from build123d import *

# Parameters (mm, degrees)
SKETCH1_W           = 60
SKETCH1_H           = 40
BOSS_EXTRUDE1_DEPTH = 10
SKETCH2_W           = 2.909575839
SKETCH2_H           = 3.168204802
CUT_EXTRUDE1_DEPTH  = 10
SKETCH3_W           = 61.747665015
SKETCH3_H           = 0.72949372
CUT_EXTRUDE2_DEPTH  = 2


with BuildPart() as part:
    # Sketch1 → Boss-Extrude1 (new body)
    with BuildSketch(Plane.XY):
        with Locations((1.914893617, 6.489361702)):
            Rectangle(SKETCH1_W, SKETCH1_H)
    extrude(amount=BOSS_EXTRUDE1_DEPTH)

    # Sketch2 → Cut-Extrude1 (cut)
    with BuildSketch(Plane.XY.offset(10)):
        with Locations((-13.721702382, 21.942442266)):
            Rectangle(SKETCH2_W, SKETCH2_H)
        with Locations((-23.721702382, 21.942442266)):
            Rectangle(SKETCH2_W, SKETCH2_H)
        with Locations((-3.721702382, 21.942442266)):
            Rectangle(SKETCH2_W, SKETCH2_H)
        with Locations((6.278297618, 21.942442266)):
            Rectangle(SKETCH2_W, SKETCH2_H)
        with Locations((16.278297619, 21.942442266)):
            Rectangle(SKETCH2_W, SKETCH2_H)
        with Locations((26.278297619, 21.942442266)):
            Rectangle(SKETCH2_W, SKETCH2_H)
        with Locations((-13.721702382, 11.942442266)):
            Rectangle(SKETCH2_W, SKETCH2_H)
        with Locations((-3.721702382, 11.942442266)):
            Rectangle(SKETCH2_W, SKETCH2_H)
        with Locations((6.278297618, 11.942442266)):
            Rectangle(SKETCH2_W, SKETCH2_H)
        with Locations((16.278297619, 11.942442266)):
            Rectangle(SKETCH2_W, SKETCH2_H)
        with Locations((26.278297619, 11.942442266)):
            Rectangle(SKETCH2_W, SKETCH2_H)
        with Locations((-13.721702382, 1.942442266)):
            Rectangle(SKETCH2_W, SKETCH2_H)
        with Locations((-3.721702382, 1.942442266)):
            Rectangle(SKETCH2_W, SKETCH2_H)
        with Locations((6.278297618, 1.942442266)):
            Rectangle(SKETCH2_W, SKETCH2_H)
        with Locations((16.278297619, 1.942442266)):
            Rectangle(SKETCH2_W, SKETCH2_H)
        with Locations((26.278297619, 1.942442266)):
            Rectangle(SKETCH2_W, SKETCH2_H)
        with Locations((-13.721702382, -8.057557734)):
            Rectangle(SKETCH2_W, SKETCH2_H)
        with Locations((-3.721702382, -8.057557734)):
            Rectangle(SKETCH2_W, SKETCH2_H)
        with Locations((6.278297618, -8.057557734)):
            Rectangle(SKETCH2_W, SKETCH2_H)
        with Locations((16.278297619, -8.057557734)):
            Rectangle(SKETCH2_W, SKETCH2_H)
        with Locations((26.278297619, -8.057557734)):
            Rectangle(SKETCH2_W, SKETCH2_H)
        with Locations((-23.721702382, 11.942442266)):
            Rectangle(SKETCH2_W, SKETCH2_H)
        with Locations((-23.721702382, 1.942442266)):
            Rectangle(SKETCH2_W, SKETCH2_H)
        with Locations((-23.721702382, -8.057557734)):
            Rectangle(SKETCH2_W, SKETCH2_H)
    extrude(amount=-CUT_EXTRUDE1_DEPTH, mode=Mode.SUBTRACT)

    # Sketch3 → Cut-Extrude2 (cut)
    with BuildSketch(Plane.XY.offset(10)):
        with Locations((1.945695922, 6.927829606)):
            Rectangle(SKETCH3_W, SKETCH3_H)
    extrude(amount=-CUT_EXTRUDE2_DEPTH, mode=Mode.SUBTRACT)


solid = part.part
Design review of the part built by this model. Coordinates are the model's own, in mm. A direction names the side the tool comes from. Give positions to 0.01 mm unless a question says otherwise; leave off trailing zeros. Order: outer loops, then holes, each group sorted by start corner. A loop starts at its lowest first (then second) coordinate and runs counter-clockwise, first axis right, second up. Notation, with made-up numbers: (-22.75, 30) - (-10.75, 30) arc R23 cw to (-10.75, 47) - close; hole circle Ø11 at (70.5, 52.25). An arc over 180 degrees is marked (long way). Use CSV: the item, a comma, the result in double quotes. Start each with the question number.
Q1. Take a section at C-C (z = 9). Count the separate pieces of the cut face and the enclosed holes in it, and give its area (4 significant figures).
Q2. Take a section at A-A (x = -24). State the section outline as (y, z) points, and give its area (3 significant figures).
Q3. For line 1 (Y direction, x = 5.5, z = 5.75); line 2 (Y direction, x = -21.5, z = 9); line 3 (Y direction, x = -14.5, z = 9), list the stretches that pass through material, from the lowest coordinate up.
Q4. Draft analysis for pull direction X (two halves, no side actions). For faces 3 (the face through (-28.085, 6, 5)), 4 (the face through (1, -3, 10)), 5 (the face through (16, 23.527, 5)), state which applies: pulls with the +X half, pulls with the -X half, needs draft (parallel to the pull), parting line crosses it, or undercut.
Q5. Take a section at B-B (y = 22.5). State the section outline as (x, z) points.
Q6. Machinability: for faces 1 (the face through (1, 17, 10)), 2 (the face through (-24, 0.358, 5)), which of the approach directions +Z, -Z, +X, -X, +Y, -Y give a long, thin tool a straight path to every point of the face, cutting with its end or side? Answer none if there is none.
Calculated:
1,separate pieces,"2"
1,enclosed holes,"24"
1,area,"2,135 mm²"
2,outline,"(-13.51, 0) - (-9.64, 0) - (-9.64, 10) - (-13.51, 10) - close; (-6.47, 0) - (0.36, 0) - (0.36, 10) - (-6.47, 10) - close; (3.53, 0) - (10.36, 0) - (10.36, 10) - (7.29, 10) - (7.29, 8) - (6.56, 8) - (6.56, 10) - (3.53, 10) - close; (13.53, 0) - (20.36, 0) - (20.36, 10) - (13.53, 10) - close; (23.53, 0) - (26.49, 0) - (26.49, 10) - (23.53, 10) - close"
2,area,"272 mm²"
3,line 1,"y = -13.51 to -9.64, -6.47 to 0.36, 3.53 to 10.36, 13.53 to 20.36, 23.53 to 26.49"
3,line 2,"y = -13.51 to 6.56, 7.29 to 26.49"
3,line 3,"y = -13.51 to -9.64, -6.47 to 0.36, 3.53 to 6.56, 7.29 to 10.36, 13.53 to 20.36, 23.53 to 26.49"
4,face 3,"pulls with the -X half"
4,face 4,"needs draft"
4,face 5,"undercut"
5,outline,"(-28.09, 0) - (-25.18, 0) - (-25.18, 10) - (-28.09, 10) - close; (-22.27, 0) - (-15.18, 0) - (-15.18, 10) - (-22.27, 10) - close; (-12.27, 0) - (-5.18, 0) - (-5.18, 10) - (-12.27, 10) - close; (-2.27, 0) - (4.82, 0) - (4.82, 10) - (-2.27, 10) - close; (7.73, 0) - (14.82, 0) - (14.82, 10) - (7.73, 10) - close; (17.73, 0) - (24.82, 0) - (24.82, 10) - (17.73, 10) - close; (27.73, 0) - (31.91, 0) - (31.91, 10) - (27.73, 10) - close"
6,face 1,"+Z, +X, -X, +Y, -Y"
6,face 2,"+Z, -Z"
